The model under review builds one solid part; all positions refer to its coordinate system, in mm. Face numbers are marked on the shaded views. A direction names the side the tool comes from. Round coordinates to 2 decimals unless told otherwise and drop trailing zeros. Write each loop counter-clockwise with the first axis right and the second up, starting at its lowest first coordinate (ties: lowest second). Pieces come first, ordered by that corner, then holes. Notation, with made-up numbers: (-26.5, 30) -> (-19.5, 30) arc R27 cw to (-19.5, 57) -> close; hole circle Ø3 at (12.25, 6). An arc over 180 degrees is marked (long way). Return JSON: item names as keys, results as strings. Group by question number.
1. For line 1 along Y through (x, z) = (-379, -16.5); line 2 along X through (y, z) = (139, -23.75); line 3 along Y through (x, z) = (-403, -31), list the stretches that pass through material, from the lowest coordinate up. Write a range as from..to.
2. Take a section at A-A, the plane x = -419.5. Write out the cut boundary in (y, z).
3. Clearance check with flat-ended pins moving along their axes: P1, Ø5, axis at x = -500.5, y = 139, coming from the -Z side; P2, Ø10, axis at y = 99, z = -28.5, coming from the -X side; P3, Ø0.5, axis at y = 199, z = -26, coming from the +X side; P4, Ø2.5, axis at y = 129, z = -16.5, coming from the +X side. State where each tip first meets the part, or that it passes through.
4. Take a section at B-B, the plane z = -23.5. Give the number of separate pieces and of enclosed holes in the cut face, then the cut area to 3 significant figures.
5. Mouldability with a two-part tool opening along Y and no side actions: class the marked faces 6, 7, 8 and 9 as pulls with the +Y half, pulls with the -Y half, needs draft (parallel to the pull), parting line crosses it, or undercut.
6. Take a section at C-C, the plane y = 83. Write out the cut boundary in (x, z).
7. Tool access review of the marked faces 1, 2, 3, 4 and 5: name each direction out of +Z, -Z, +X, -X, +Y, -Y from which nothing blocks a thin tool from reaching the whole face with its end or side.
Autodesk Inventor part; units mm, degrees
ref_plane "YZ Plane" through (0, 0, 0) normal (1, 0, 0) x (0, 1, 0)
ref_plane "XZ Plane" through (0, 0, 0) normal (0, 1, 0) x (-1, 0, 0)
ref_plane "XY Plane" through (0, 0, 0) normal (0, 0, 1) x (1, 0, 0)
ref_plane "Work Plane1" through (-191.4749, 128.3402, -15) normal (0, 0, -1) x (-1, 0, 0)
sketch "Sketch1" plane through (-191.4749, 128.3402, -15) normal (0, 0, -1) x (-1, 0, 0)
  line L0 (190.8, 9) -> (190.8, -9) construction
  line L1 (221.5, 38.1385) -> (221.5, 59.5385) construction
  line L2 (228.2, 37.8385) -> (228.2, 59.8385) construction
  line L3 (292.4096, 87.8385) -> (292.4096, -112.1615) construction
  line L4 (308.2846, 87.8385) -> (308.2846, -112.1615) construction
  line L5 (240.5, -40) -> (240.5, 20.35)
  line L6 (240.5, 20.35) -> (277.4096, 20.35)
  line L7 (277.4096, 20.35) -> (277.4096, 6.35)
  line L8 (277.4096, 6.35) -> (328.2846, 6.35)
  line L9 (328.2846, 6.35) -> (328.2846, -6.35)
  line L10 (328.2846, -6.35) -> (272.4096, -6.35)
  line L11 (272.4096, -6.35) -> (272.4096, -65)
  line L12 (272.4096, -65) -> (165.5, -65)
  line L13 (165.5, -65) -> (165.5, 60.1385)
  line L14 (165.5, 60.1385) -> (220.5, 60.1385)
  line L15 (220.5, 60.1385) -> (220.5, 40.1385)
  line L16 (220.5, 40.1385) -> (190.5, 40.1385)
  line L17 (190.5, 40.1385) -> (206.5, 40.1385)
  line L18 (206.5, 40.1385) -> (206.5, 30.1385)
  line L19 (206.5, 30.1385) -> (190.5, 30.1385)
  line L20 (190.5, 30.1385) -> (190.5, 40.1385)
  line L21 (190.5, 30.1385) -> (190.5, -40)
  line L22 (190.5, -40) -> (240.5, -40)
  line L23 (190.5, -8.7) -> (190.5, 8.7) construction
  point P0 (-191.4749, -128.3402)
  point P1 (328.2846, 0)
  point P2 (190.8, 0)
  point P3 (190.5, 0)
  dimension "d0" = 12.7
  dimension "d1" = 2
  dimension "d2" = 1
  dimension "d3" = 20
  dimension "d4" = 16
  dimension "d5" = 10
  dimension "d6" = 40
  dimension "d7" = 25
  dimension "d8" = 50
  dimension "d9" = 20
  dimension "d10" = 20
  dimension "d11" = 15
  dimension "d12" = 14
  dimension "d13" = 25
extrude "Extrusion1" add sketch "Sketch1" along normal blind 20
sketch "Sketch2" plane through (-519.7595, 121.9902, -15) normal (0, -1, 0) x (1, 0, 0)
  circle A0 centre (27.9375, 0) radius 30 construction
  circle A1 centre (27.9375, 0) radius 17.4625
  point P0 (519.7595, 15)
  dimension "d16" = 34.925
extrude "Extrusion2" cut sketch "Sketch2" against normal through all
sketch "Sketch3" plane through (-191.4749, 128.3402, -15) normal (0, 0, 1) x (1, 0, 0)
  line L0 (-317.8096, -6.35) -> (-317.8096, 6.35)
  line L1 (-333.8096, 8) -> (-317.8096, 8)
  line L2 (-317.8096, 8) -> (-317.8096, -8)
  line L3 (-317.8096, -8) -> (-333.8096, -8)
  line L4 (-333.8096, -8) -> (-333.8096, 8)
  point P0 (191.4749, -128.3402)
  point P1 (-317.8096, 0)
  dimension "d19" = 16
  dimension "d20" = 16
extrude "Extrusion3" add sketch "Sketch3" against normal up to surface (20 mm away)
sketch "Sketch4" plane through (-191.4749, 128.3402, -35) normal (0, 0, -1) x (-1, 0, 0)
  line L0 (317.8096, -8) -> (333.8096, -8)
  line L1 (333.8096, 8) -> (317.8096, 8)
  line L2 (325.8096, 8) -> (325.8096, -8)
  circle A0 centre (325.8096, 0) radius 4
  point P0 (-191.4749, -128.3402)
  dimension "d23" = 8
extrude "Extrusion4" cut sketch "Sketch4" against normal through all
sketch "Sketch5" plane through (-356.9749, 63.3402, -15) normal (1, 0, 0) x (0, 0, -1)
  arc A0 (1.3364, 96.1329) -> (-1.3364, 96.1329) centre (0, 65) ccw construction
  arc A1 (-1.3364, 96.1329) -> (-7.1127, 95.3389) centre (0, 65) ccw construction
  arc A2 (-7.1127, 95.3389) -> (-9.6864, 94.6178) centre (0, 65) ccw construction
  arc A3 (-9.6864, 94.6178) -> (-15.0343, 92.2949) centre (0, 65) ccw construction
  arc A4 (-15.0343, 92.2949) -> (-17.318, 90.9062) centre (0, 65) ccw construction
  arc A5 (-17.318, 90.9062) -> (-21.8409, 87.2265) centre (0, 65) ccw construction
  arc A6 (-21.8409, 87.2265) -> (-23.6652, 85.2731) centre (0, 65) ccw construction
  arc A7 (-23.6652, 85.2731) -> (-27.0276, 80.5097) centre (0, 65) ccw construction
  arc A8 (-27.0276, 80.5097) -> (-28.2572, 78.1366) centre (0, 65) ccw construction
  arc A9 (-28.2572, 78.1366) -> (-30.2098, 72.6426) centre (0, 65) ccw construction
  arc A10 (-30.2098, 72.6426) -> (-30.7536, 70.0257) centre (0, 65) ccw construction
  arc A11 (-30.7536, 70.0257) -> (-31.1515, 64.2087) centre (0, 65) ccw construction
  arc A12 (-31.1515, 64.2087) -> (-30.9691, 61.5421) centre (0, 65) ccw construction
  arc A13 (-30.9691, 61.5421) -> (-29.7828, 55.8335) centre (0, 65) ccw construction
  arc A14 (-29.7828, 55.8335) -> (-28.8878, 53.315) centre (0, 65) ccw construction
  arc A15 (-28.8878, 53.315) -> (-26.2053, 48.1381) centre (0, 65) ccw construction
  arc A16 (-26.2053, 48.1381) -> (-24.6639, 45.9545) centre (0, 65) ccw construction
  arc A17 (-24.6639, 45.9545) -> (-20.6842, 41.6933) centre (0, 65) ccw construction
  arc A18 (-20.6842, 41.6933) -> (-18.6109, 40.0065) centre (0, 65) ccw construction
  arc A19 (-18.6109, 40.0065) -> (-13.6291, 36.977) centre (0, 65) ccw construction
  arc A20 (-13.6291, 36.977) -> (-11.1776, 35.9122) centre (0, 65) ccw construction
  arc A21 (-11.1776, 35.9122) -> (-5.5632, 34.3391) centre (0, 65) ccw construction
  arc A22 (-5.5632, 34.3391) -> (-2.9153, 33.9751) centre (0, 65) ccw construction
  arc A23 (-2.9153, 33.9751) -> (2.9153, 33.9751) centre (0, 65) ccw construction
  arc A24 (2.9153, 33.9751) -> (5.5632, 34.3391) centre (0, 65) ccw construction
  arc A25 (5.5632, 34.3391) -> (11.1776, 35.9122) centre (0, 65) ccw construction
  arc A26 (11.1776, 35.9122) -> (13.6291, 36.977) centre (0, 65) ccw construction
  arc A27 (13.6291, 36.977) -> (18.6109, 40.0065) centre (0, 65) ccw construction
  arc A28 (18.6109, 40.0065) -> (20.6842, 41.6933) centre (0, 65) ccw construction
  arc A29 (20.6842, 41.6933) -> (24.6639, 45.9545) centre (0, 65) ccw construction
  arc A30 (24.6639, 45.9545) -> (26.2053, 48.1381) centre (0, 65) ccw construction
  arc A31 (26.2053, 48.1381) -> (28.8878, 53.315) centre (0, 65) ccw construction
  arc A32 (28.8878, 53.315) -> (29.7828, 55.8335) centre (0, 65) ccw construction
  arc A33 (29.7828, 55.8335) -> (30.9691, 61.5421) centre (0, 65) ccw construction
  arc A34 (30.9691, 61.5421) -> (31.1515, 64.2087) centre (0, 65) ccw construction
  arc A35 (31.1515, 64.2087) -> (30.7536, 70.0257) centre (0, 65) ccw construction
  arc A36 (30.7536, 70.0257) -> (30.2098, 72.6426) centre (0, 65) ccw construction
  arc A37 (30.2098, 72.6426) -> (28.2572, 78.1366) centre (0, 65) ccw construction
  arc A38 (28.2572, 78.1366) -> (27.0276, 80.5097) centre (0, 65) ccw construction
  arc A39 (27.0276, 80.5097) -> (23.6652, 85.2731) centre (0, 65) ccw construction
  arc A40 (23.6652, 85.2731) -> (21.8409, 87.2265) centre (0, 65) ccw construction
  arc A41 (21.8409, 87.2265) -> (17.318, 90.9062) centre (0, 65) ccw construction
  arc A42 (17.318, 90.9062) -> (15.0343, 92.2949) centre (0, 65) ccw construction
  arc A43 (15.0343, 92.2949) -> (9.6864, 94.6178) centre (0, 65) ccw construction
  arc A44 (9.6864, 94.6178) -> (7.1127, 95.3389) centre (0, 65) ccw construction
  arc A45 (7.1127, 95.3389) -> (1.3364, 96.1329) centre (0, 65) ccw construction
  circle A46 centre (-10, 65) radius 3 construction
  arc A47 (7, 65) -> (-7, 65) centre (0, 65) ccw construction
  circle A48 centre (10, 65) radius 3 construction
  arc A49 (-7, 65) -> (7, 65) centre (0, 65) ccw construction
  circle A50 centre (0, 65) radius 5
  point P0 (-15, -63.3402)
  dimension "d26" = 10
extrude "Extrusion5" cut sketch "Sketch5" against normal blind 95
sketch "Sketch6" plane through (-431.9749, 88.3402, -35) normal (1, 0, 0) x (0, 0, -1)
  arc A0 (-20, 35) -> (-20, 45) centre (-20, 40) ccw
  circle A1 centre (-20, 40) radius 11
  point P0 (-35, -88.3402)
  dimension "d29" = 22
extrude "Extrusion6" cut sketch "Sketch6" against normal blind 7
sketch "Sketch7" plane through (-356.9749, 63.3402, -35) normal (1, 0, 0) x (0, 0, -1)
  arc A0 (-20, 60) -> (-20, 70) centre (-20, 65) ccw
  circle A1 centre (-20, 65) radius 11
  point P0 (-35, -63.3402)
  dimension "d32" = 22
extrude "Extrusion7" cut sketch "Sketch7" against normal blind 15
sketch "Sketch8" plane through (-191.4749, 128.3402, -35) normal (0, 0, -1) x (-1, 0, 0)
  line L0 (220.5, 60.1385) -> (204.5, 60.1385)
  line L1 (204.5, 60.1385) -> (204.5, 76.1385)
  line L2 (204.5, 76.1385) -> (220.5, 76.1385)
  line L3 (220.5, 76.1385) -> (220.5, 60.1385)
  point P0 (-191.4749, -128.3402)
  dimension "d35" = 16
  dimension "d36" = 16
extrude "Extrusion8" add sketch "Sketch8" against normal up to surface (20 mm away)
sketch "Sketch9" plane through (-356.9749, 63.3402, -35) normal (1, 0, 0) x (0, 0, -1)
  circle A0 centre (-20, 113.8385) radius 10.7
  circle A1 centre (-20, 113.8385) radius 10.7
  circle A2 centre (-20, 113.8385) radius 4
  point P0 (-35, -63.3402)
  dimension "d39" = 8
extrude "Extrusion9" cut sketch "Sketch9" against normal through all contours A2
sketch "Sketch10" plane through (-191.4749, 128.3402, -35) normal (0, 0, -1) x (-1, 0, 0)
  line L0 (277.4096, 6.35) -> (277.4096, 20.35)
  line L1 (190.5, 30.1385) -> (206.5, 30.1385)
  line L2 (220.5, 40.1385) -> (220.5, 76.1385)
  line L3 (204.5, 76.1385) -> (204.5, 60.1385)
  line L4 (165.5, 60.1385) -> (165.5, -65)
  line L5 (165.5, -65) -> (272.4096, -65)
  line L6 (204.5, 68.1385) -> (220.5, 68.1385) construction
  line L7 (198.5, 30.1385) -> (198.5, 40.1385) construction
  line L8 (198.5, 40.1385) -> (206.5, 40.1385) construction
  circle A0 centre (198.5, 40.1385) radius 4
  circle A1 centre (212.5, 68.1385) radius 4
  line L9 (247.5, 11) -> (240.5, 11) construction
  line L10 (240.5, -11) -> (247.5, -11) construction
  line L11 (247.5, 11) -> (247.5, -11) construction
  line L12 (282.8846, 6.35) -> (282.8846, -6.35) construction
  line L13 (247.5, 0) -> (255.5, 0) construction
  line L14 (255.5, 12.5) -> (255.5, -12.5) construction
  line L15 (260.5, 5) -> (247.5, 5) construction
  line L16 (247.5, -5) -> (260.5, -5) construction
  circle A2 centre (255.5, 12.5) radius 4
  circle A3 centre (255.5, -12.5) radius 4
  line L17 (180.5, -53) -> (257.4096, -53) construction
  circle A4 centre (180.5, -53) radius 4
  circle A5 centre (257.4096, -53) radius 4
  line L18 (272.4096, -65) -> (272.4096, -6.35)
  line L19 (180.5, -5) -> (190.5, -5) construction
  line L20 (190.5, 5) -> (180.5, 5) construction
  line L21 (180.5, 11) -> (165.5, 11) construction
  line L22 (165.5, -11) -> (180.5, -11) construction
  line L23 (175.5, 20) -> (175.5, -20) construction
  circle A6 centre (175.5, 20) radius 4
  circle A7 centre (175.5, -20) radius 4
  line L24 (165.5, -11) -> (165.5, 11)
  point P0 (-191.4749, -128.3402)
  point P1 (175.5, 0)
  point P2 (165.5, 0)
  dimension "d42" = 8
  dimension "d43" = 8
  dimension "d46" = 8
  dimension "d47" = 25
  dimension "d48" = 8
  dimension "d49" = 8
  dimension "d50" = 12
  dimension "d51" = 15
  dimension "d52" = 15
  dimension "d53" = 8
  dimension "d54" = 40
  dimension "d55" = 10
extrude "Extrusion10" cut sketch "Sketch10" against normal through all
chamfer "Chamfer1" distance 5 angle 45 2 edges at (-397.9749, 168.4787, -25) (-397.9749, 158.4787, -25)
chamfer "Chamfer2" distance 10 angle 45 2 edges at (-395.9749, 188.4787, -25) (-381.9749, 158.4787, -25)
chamfer "Chamfer3" distance 5 angle 45 3 edges at (-395.9749, 204.4787, -25) (-411.9749, 204.4787, -25) (-411.9749, 168.4787, -25)
chamfer "Chamfer4" distance 5 angle 45 1 edges at (-356.9749, 188.4787, -25)
chamfer "Chamfer5" distance 10 angle 45 2 edges at (-356.9749, 63.3402, -25) (-463.8845, 63.3402, -25)
chamfer "Chamfer6" distance 10 angle 45 2 edges at (-381.9749, 88.3402, -25) (-431.9749, 88.3402, -25)
chamfer "Chamfer7" distance 10 angle 45 2 edges at (-468.8845, 148.6902, -25) (-463.8845, 121.9902, -25)
chamfer "Chamfer8" distance 5 angle 45 1 edges at (-431.9749, 148.6902, -25)
properties part number "gear frame 1"
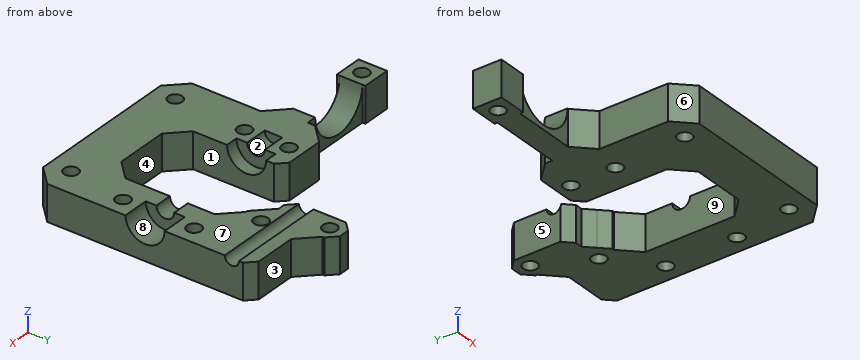
Output:
{
 "1": {"line 1": "y = 63.34..123.57, 133.11..173.47, 180.89..188.48", "line 2": "x = -468.57..-450.53, -443.42..-431.97, -381.97..-356.97", "line 3": "y = 63.34..88.34, 168.48..192.6, 200.36..204.48"},
 "2": {"outline": "(63.34, -35) -> (88.34, -35) -> (88.34, -15) -> (63.34, -15) -> close"},
 "3": {"P1": "passes through", "P2": "stops at x = -463.88", "P3": "stops at x = -395.97", "P4": "stops at x = -451.97"},
 "4": {"separate pieces": "2", "enclosed holes": "9", "area": "7,910 mm^2"},
 "5": {"face 6": "pulls with the -Y half", "face 7": "needs draft", "face 8": "undercut", "face 9": "undercut"},
 "6": {"outline": "(-463.88, -35) -> (-356.97, -35) -> (-356.97, -15) -> (-463.88, -15) -> close"},
 "7": {"face 1": "+Z, -Z, +Y", "face 2": "+Z, +X", "face 3": "+Z, -Z, +X, +Y", "face 4": "+Z, -Z", "face 5": "+Z, -Z, -X, +Y"}
}
